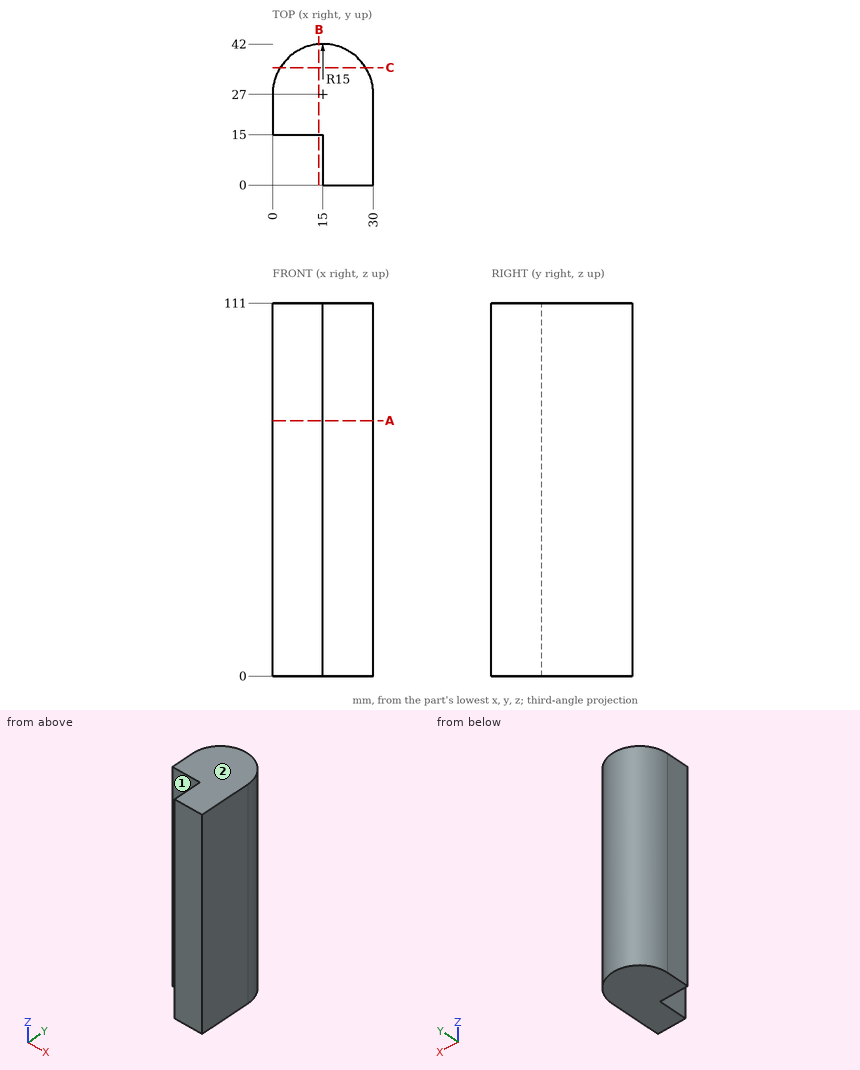
Input: dimensioned drawing with shaded views. Units: mm. Origin: part minimum x, y, z. A direction names the side the tool comes from. Give positions to 0.01 mm unless a question says otherwise; leave off trailing zeros. Loops run counter-clockwise (first coordinate to the right, second up) from the corner with the lowest first, then second, coordinate; pieces in that order, holes last. Notation, with made-up numbers: M 57,61.5 L 84,61.5 A19 ccw 84,81.5 Z; hole C -5,58.5 d9. An arc over 180 degrees is marked long. Put each result on its own line as item: value.
1) First-contact query: P1, Ø1, axis at y = 32, z = 17, coming from the +X side; P2, Ø7.5, axis at y = 8, z = 67.5, coming from the -X side; P3, Ø1.5, axis at y = 35.5, z = 95.5, coming from the -X side. Flat tips, straight axial feed; report the tip coordinate or a pass-through.
Computed values:
P1: stops at x = 29.31
P2: stops at x = 15
P3: stops at x = 2.16
2) Cut plane B-B, the plane x = 13.75. Return the cut outline in (y, z), plus the area to 3 significant figures.
Computed values:
outline: M 15,0 L 41.95,0 L 41.95,111 L 15,111 Z
area: 2,990 mm^2
3) Cut plane C-C, the plane y = 35. Return the cut outline in (x, z), plus the area to 3 significant figures.
Computed values:
outline: M 2.31,0 L 27.69,0 L 27.69,111 L 2.31,111 Z
area: 2,820 mm^2
4) Reachability of the marked faces 1 and 2 from +Z, -Z, +X, -X, +Y, -Y: full face, straight path, thin tool, end or side. Return the list, or none.
Computed values:
face 1: +Z, -Z, -X, -Y
face 2: +Z, +X, -X, +Y, -Y
5) Material intervals for L1, parallel to X at y = 11, z = 18; L2, parallel to X at y = 34, z = 103; L3, parallel to Y at x = 5.75, z = 103, sorted ascending. Write a range as from..to.
Computed values:
L1: x = 15..30
L2: x = 1.73..28.27
L3: y = 15..38.81
6) Cut plane A-A, the plane z = 76. Return the cut outline in (x, y).
Computed values:
outline: M 0,15 L 15,15 L 15,0 L 30,0 L 30,27 A15 ccw 0,27 Z
